Autodesk Fusion 360 part; units mm, degrees
sketch "Sketch1" plane through (0, 0, 0) normal (0, 0, 1) x (1, 0, 0)
  circle A0 centre (0, 0) radius 12.7
  circle A1 centre (0, 0) radius 2.7781
  dimension "d1" = 25.4
  dimension "d2" = 5.5563
extrude "Extrude1" add sketch "Sketch1" along normal blind 3.81
sketch "Sketch2" plane through (0, 0, 3.81) normal (0, 0, 1) x (-1, 0, 0)
  circle A0 centre (0, 0) radius 2.7781
  circle A1 centre (0, 0) radius 12.7
  circle A2 centre (0, 0) radius 2.7781
  circle A3 centre (0, 0) radius 6.35
  line L0 (0, 0) -> (0, -12.7) construction
  line L1 (0, 0) -> (0, 12.7) construction
  line L2 (0, 0) -> (-12.7, 0) construction
  line L3 (0, 0) -> (12.7, 0) construction
  circle A4 centre (0, 0) radius 9.525 construction
  circle A5 centre (0, -9.525) radius 1.5
  arc A6 (-8.2489, 4.7625) -> (0, -9.525) centre (0, 0) ccw construction
  line L4 (0, 0) -> (-8.2489, 4.7625) construction
  line L5 (0, 0) -> (0, -9.525) construction
  arc A7 (0, -9.525) -> (8.2489, 4.7625) centre (0, 0) ccw construction
  line L6 (0, 0) -> (0, -9.525) construction
  line L7 (0, 0) -> (8.2489, 4.7625) construction
  circle A8 centre (-8.2489, 4.7625) radius 1.5
  circle A9 centre (8.2489, 4.7625) radius 1.5
  dimension "d5" = 5.5563
  dimension "d6" = 12.7
  dimension "d9" = 19.05
  dimension "d10" = 3
  dimension "d11" = 120
  dimension "d12" = 120
  dimension "d13" = 3
  dimension "d14" = 3
extrude "Extrude3" cut sketch "Sketch2" against normal blind 3.81 contours A5 | A8 | A9
extrude "Extrude2" add sketch "Sketch2" along normal blind 15.24 contours A3
equation "d7 = 19.05 mm - 3.81 mm"
Read the model definition and answer for the solid it produces. Units are mm, in the model's axes. A direction names the side the tool comes from. Give positions to 0.01 mm unless a question says otherwise; leave off trailing zeros. Order: outer loops, then holes, each group sorted by start corner. A loop starts at its lowest first (then second) coordinate and runs counter-clockwise, first axis right, second up. Notation, with made-up numbers: (2, -14) -> (7, -14) arc R13 cw to (7, 8) -> close; hole circle Ø10 at (62.25, 9.25). An arc over 180 degrees is marked (long way). Write item = value, one per line.
1. A cutting plane is placed at D-D, the plane z = 15.75. Write down the section's boundary in (x, y).
Numbers:
outline = circle Ø12.7 at (0, 0); hole circle Ø5.56 at (0, 0)
2. For faces 4 (the face through (-2.75, 12.4, 1.88)), 5 (the face through (3, 6, 3.81)), determine the directions among +Z, -Z, +X, -X, +Y, -Y from which every point of the face is accessible in a straight line to the end or side of a thin tool.
Numbers:
face_4 = +Z, -Z
face_5 = +Z
3. The mould has two halves that part along Y. Classify faces 1 (the face through (0, 3, 0)), 2 (the face through (1.38, -6.2, 11.32)), 3 (the face through (0.2, 8.04, 1.93)): +Y half, -Y half, draft (parallel to the pull), parting line (faces both ways), or undercut.
Numbers:
face_1 = draft
face_2 = parting line
face_3 = undercut
4. Given pin 1 (2 mm diameter, centred on y = 6, z = 8, fed in from +X); pin 2 (9 mm diameter, centred on x = 0, y = 0, fed in from -Z); pin 3 (5 mm diameter, centred on x = 3.5, z = 10, fed in from +Y); pin 4 (1.5 mm diameter, centred on x = 5, y = -8, fed in from +Z), each flat-ended and moving along its own axis, determine where each tip first touches the part or whether it passes through.
Numbers:
pin_1 = 3.91
pin_2 = 0
pin_3 = 6.27
pin_4 = 3.81
5. A cutting plane is placed at B-B, the plane x = 0. Write down the section's boundary in (y, z) (3 decimals), and give its area (3 significant figures).
Numbers:
outline = (-12.7, 0) -> (-2.778, 0) -> (-2.778, 19.05) -> (-6.35, 19.05) -> (-6.35, 3.81) -> (-12.7, 3.81) -> close; (2.778, 0) -> (8.025, 0) -> (8.025, 3.81) -> (6.35, 3.81) -> (6.35, 19.05) -> (2.778, 19.05) -> close; (11.025, 0) -> (12.7, 0) -> (12.7, 3.81) -> (11.025, 3.81) -> close
area = 173 mm²
6. A cutting plane is placed at C-C, the plane y = -4.25. Write down the section's boundary in (x, z).
Numbers:
outline = (-11.97, 0) -> (-9.66, 0) -> (-9.66, 3.81) -> (-11.97, 3.81) -> close; (-6.84, 0) -> (6.84, 0) -> (6.84, 3.81) -> (4.72, 3.81) -> (4.72, 19.05) -> (-4.72, 19.05) -> (-4.72, 3.81) -> (-6.84, 3.81) -> close; (9.66, 0) -> (11.97, 0) -> (11.97, 3.81) -> (9.66, 3.81) -> close
7. Straight lines are drawn through the part: line 1 along Y through (x, z) = (0, 1.1) (3 decimals); line 2 along Z through (x, y) = (6.5, -6); line 3 along Y through (x, z) = (-7, 3). For each, find the intervals that lie inside material, in ascending order.
Numbers:
line_1 = -12.7 to -2.778, 2.778 to 8.025, 11.025 to 12.7
line_2 = 0 to 3.81
line_3 = -10.6 to -5.59, -3.93 to 10.6
8. A cutting plane is placed at A-A, the plane y = 0. Write down the section's boundary in (x, z).
Numbers:
outline = (-12.7, 0) -> (-2.78, 0) -> (-2.78, 19.05) -> (-6.35, 19.05) -> (-6.35, 3.81) -> (-12.7, 3.81) -> close; (2.78, 0) -> (12.7, 0) -> (12.7, 3.81) -> (6.35, 3.81) -> (6.35, 19.05) -> (2.78, 19.05) -> close
